from build123d import *

# Parameters (mm, degrees)
ESBO_O1_W   = 40
ESBO_O1_H   = 20
ESBO_O1_W_2 = 36
ESBO_O1_H_2 = 16


with BuildPart() as part:
    # Varredura1: sweep along a path in Esboço2
    with BuildLine(Plane(origin=(0, 0, 0), x_dir=(0, 0, -1), z_dir=(1, 0, 0))) as varredura1_path:
        Line((0, 0), (0, -400))
    # Esboço1 → Varredura1 (sweep)
    with BuildSketch(Plane(origin=(0, 0, 0), x_dir=(1, 0, 0), z_dir=(0, 1, 0))):
        Rectangle(ESBO_O1_W, ESBO_O1_H)
        Rectangle(ESBO_O1_W_2, ESBO_O1_H_2, mode=Mode.SUBTRACT)
    sweep(path=varredura1_path.line)


solid = part.part
Geometry: final body of the model. Coordinates: model frame, mm. A direction names the side the tool comes from. Give positions to 0.01 mm unless a question says otherwise; leave off trailing zeros. Write each loop counter-clockwise with the first axis right and the second up, starting at its lowest first coordinate (ties: lowest second). Pieces come first, ordered by that corner, then holes. Notation, with made-up numbers: (10, 43) - (19, 43) arc R16 ccw to (19, 68) - close; hole circle Ø11 at (64.5, -11). An arc over 180 degrees is marked (long way). Return JSON: item names as keys, results as strings. Group by question number.
1) Set-up query: faces 1 (the flat face through (-18, -203, 0)), 2 (the flat face through (0, -203, 10)). Return all of +Z, -Z, +X, -X, +Y, -Y with unobstructed straight access to the full face (end or side cutting, diameter ignored); none if empty.
2) Section A-A on z = -0.5. Return the cut outline in (x, y).
3) First-contact query: P1, Ø10, axis at x = 11, z = 4.5, coming from the -Y side. Flat tip, straight axial feed; report the tip coordinate or a pass-through.
4) Line query: line 1 (X direction, y = -201, z = 7); line 2 (Z direction, x = 17, y = -46.5). Output: solid intervals per line, ascending.
5) Mould query, pull axis Z, two halves, no side actions, for faces 3 (the flat face through (0, -203, -8)), 4 (the flat face through (0, -203, -10)), 5 (the flat face through (1.6, -400, -8.2)). Classes: released by +Z, released by -Z, zero draft, split by the parting line, or undercut.
6) Section B-B on y = -250. Return the cut outline in (x, z).
7) Section C-C on x = -3.5. Return the cut outline in (y, z), plus the area to 3 significant figures.
Filled in:
{
 "1": {"face 1": "+Y, -Y", "face 2": "+Z, +X, -X, +Y, -Y"},
 "2": {"outline": "(-20, -400) - (-18, -400) - (-18, 0) - (-20, 0) - close; (18, -400) - (20, -400) - (20, 0) - (18, 0) - close"},
 "3": {"P1": "stops at y = -400"},
 "4": {"line 1": "x = -20 to -18, 18 to 20", "line 2": "z = -10 to -8, 8 to 10"},
 "5": {"face 3": "undercut", "face 4": "released by -Z", "face 5": "zero draft"},
 "6": {"outline": "(-20, -10) - (20, -10) - (20, 10) - (-20, 10) - close; hole (-18, -8) - (18, -8) - (18, 8) - (-18, 8) - close"},
 "7": {"outline": "(-400, -10) - (0, -10) - (0, -8) - (-400, -8) - close; (-400, 8) - (0, 8) - (0, 10) - (-400, 10) - close", "area": "1,600 mm^2"}
}
